Input: dimensioned drawing with shaded views. Units: mm. Origin: part minimum x, y, z. Round coordinates to 2 decimals unless told otherwise and drop trailing zeros. Write each loop counter-clockwise with the first axis right and the second up, starting at its lowest first coordinate (ties: lowest second). Pieces come first, ordered by that corner, then holes. Notation, with made-up numbers: (38, 17.25) - (68, 17.25) arc R8 cw to (68, 22.25) - close; hole circle Ø2 at (-8, 58.25). An arc over 180 degrees is marked (long way). Use one line per item in the form item = value.
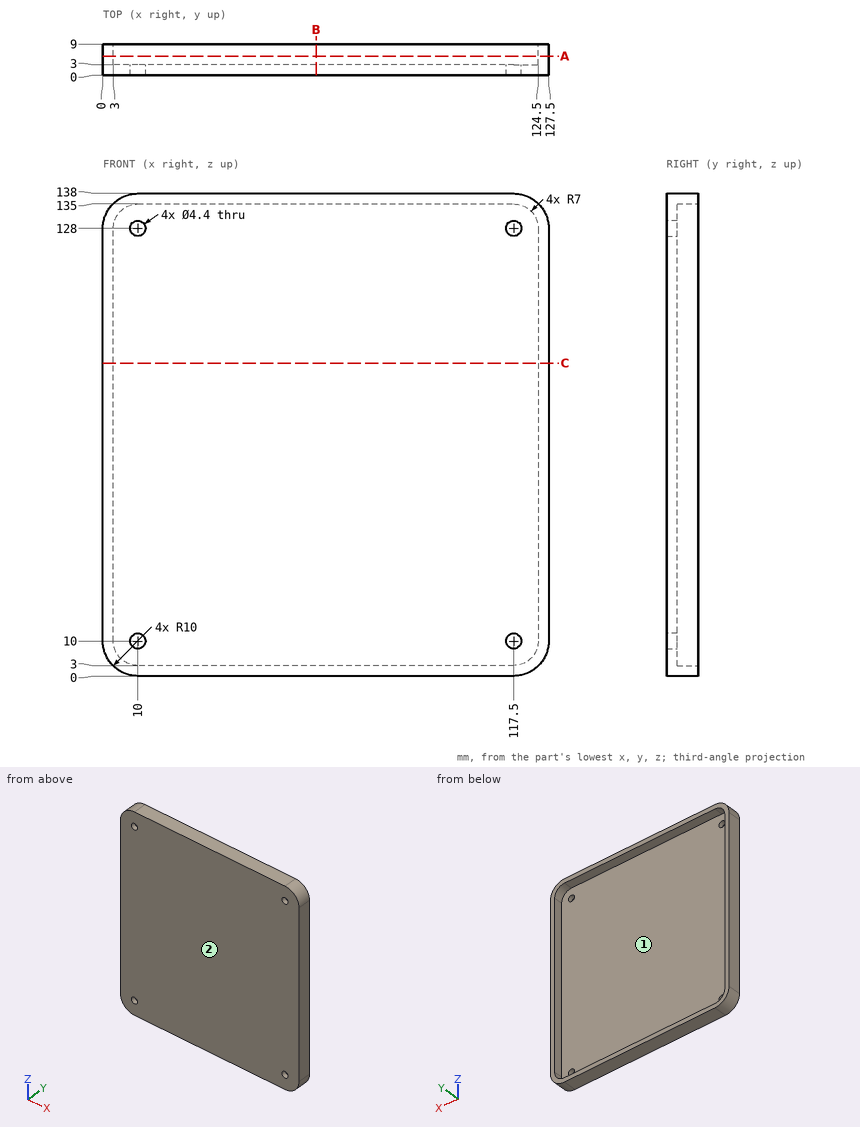
(1) First-contact query: pin 1 Ø7 at (x, z) = (117.5, 10) entering from +Y. Flat tip, straight axial feed; report the tip coordinate or a pass-through.
Derived:
pin_1 = 3
(2) Draft query along X for the marked faces 1 and 2. Return one class per face: released by +X, released by -X, zero draft, split by the parting line, or undercut.
Derived:
face_1 = undercut
face_2 = zero draft
(3) Cut plane B-B on x = 61. Output: boundary loops of the cut face in (y, z), then the cut area to 3 significant figures.
Derived:
outline = (0, 0) - (9, 0) - (9, 3) - (3, 3) - (3, 135) - (9, 135) - (9, 138) - (0, 138) - close
area = 450 mm^2
(4) Cut plane A-A on y = 5.5. Output: boundary loops of the cut face in (x, z), then the cut area to 3 significant figures.
Derived:
outline = (0, 10) arc R10 ccw to (10, 0) - (117.5, 0) arc R10 ccw to (127.5, 10) - (127.5, 128) arc R10 ccw to (117.5, 138) - (10, 138) arc R10 ccw to (0, 128) - close; hole (3, 10) arc R7 ccw to (10, 3) - (117.5, 3) arc R7 ccw to (124.5, 10) - (124.5, 128) arc R7 ccw to (117.5, 135) - (10, 135) arc R7 ccw to (3, 128) - close
area = 1,510 mm^2
(5) Material intervals for L1, parallel to X at y = 2.2, z = 10; L2, parallel to Z at x = 117.5, y = 1.4; L3, parallel to Z at x = 101, y = 7, sorted ascending.
Derived:
L1 = 0 to 7.8, 12.2 to 115.3, 119.7 to 127.5
L2 = 0 to 7.8, 12.2 to 125.8, 130.2 to 138
L3 = 0 to 3, 135 to 138
(6) Cut plane C-C on z = 89.5. Output: boundary loops of the cut face in (x, y), then the cut area to 4 significant figures.
Derived:
outline = (0, 0) - (127.5, 0) - (127.5, 9) - (124.5, 9) - (124.5, 3) - (3, 3) - (3, 9) - (0, 9) - close
area = 418.5 mm^2
